Verification items for this drawing (mm, ordinates from the low corner). A direction names the side the tool comes from. Coordinates: 2 decimals unless noted, no trailing zeros. Write each loop counter-clockwise with the first axis right and the second up, starting at its lowest first coordinate (ties: lowest second). Pieces come first, ordered by that corner, then holes. Notation, with made-up numbers: (-2.75, 10) -> (1.25, 10) arc R36 ccw to (1.25, 47) -> close; hole circle Ø2 at (-24.5, 61). An arc over 180 degrees is marked (long way). Use CSV: the item, a comma, the result in double quotes.
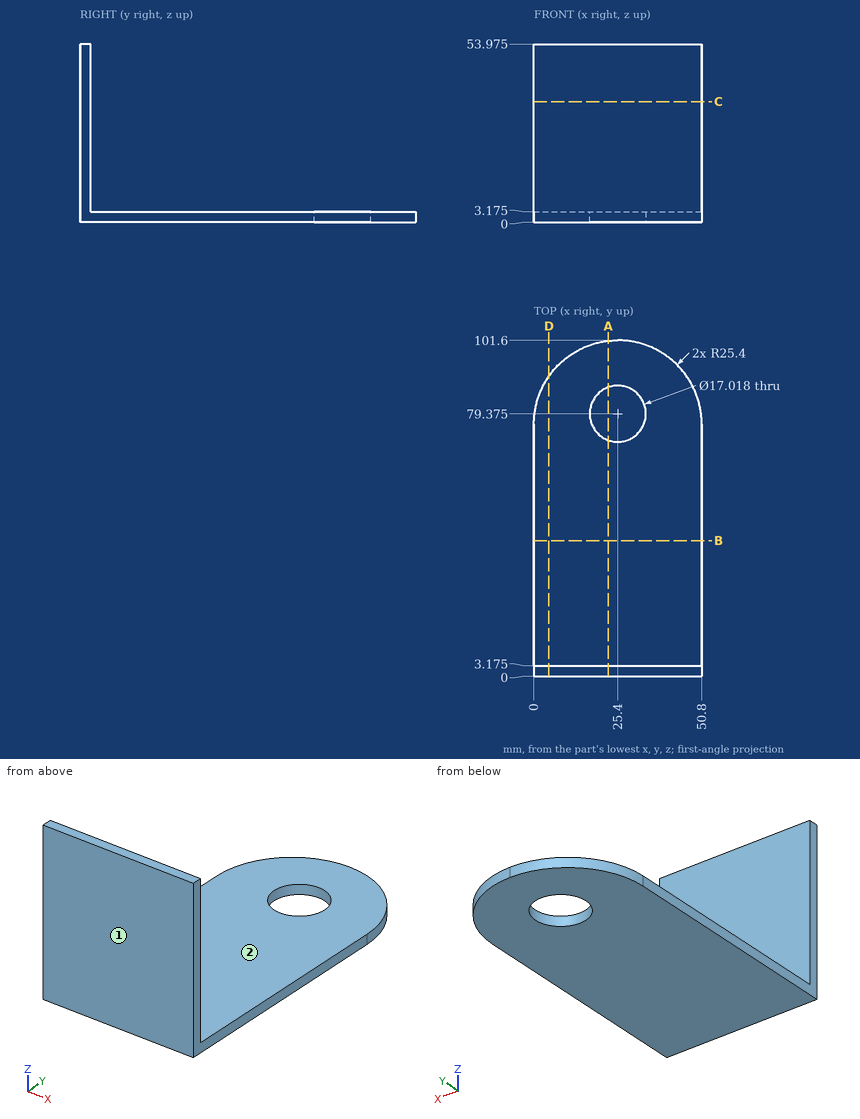
1) Cross-section at A-A (x = 22.5). Record the boundary of the cut face in (y, z) (1 decimal).
Return value:
outline,"(0, 0) -> (71.4, 0) -> (71.4, 3.2) -> (3.2, 3.2) -> (3.2, 54) -> (0, 54) -> close; (87.4, 0) -> (101.4, 0) -> (101.4, 3.2) -> (87.4, 3.2) -> close"
2) Cross-section at D-D (x = 4.5). Record the boundary of the cut face in (y, z) (1 decimal).
Return value:
outline,"(0, 0) -> (90.6, 0) -> (90.6, 3.2) -> (3.2, 3.2) -> (3.2, 54) -> (0, 54) -> close"
3) Scan lines: L1, parallel to Y at x = 25.4, z = 2.2; L2, parallel to Z at x = 47, y = 48.5 (3 decimals). Record each from-to range of solid material in increasing order.
Return value:
L1,"0 to 70.87, 87.88 to 101.6"
L2,"0 to 3.175"
4) Gauge pin test, flat ends, axial feed: pin 1 (1 mm diameter, centred on x = 45, z = 20.5, fed in from +Y) (3 decimals); pin 2 (2 mm diameter, centred on x = 19, z = 22, fed in from -Y); pin 3 (1.5 mm diameter, centred on x = 15.5, y = 77, fed in from +Z) (3 decimals). Record the tip position at first contact, or that the pin passes through.
Return value:
pin 1,"y = 3.175"
pin 2,"y = 0"
pin 3,"z = 3.175"
5) Cross-section at B-B (y = 41). Record the boundary of the cut face in (x, z) (3 decimals), plus the area to 3 significant figures.
Return value:
outline,"(0, 0) -> (50.8, 0) -> (50.8, 3.175) -> (0, 3.175) -> close"
area,"161 mm2"
6) Set-up check for the marked faces 1 and 2: record each of +Z, -Z, +X, -X, +Y, -Y from which the full face is reachable in a straight line by a thin tool's end or side.
Return value:
face 1,"+Z, -Z, +X, -X, -Y"
face 2,"+Z, +X, -X, +Y"
